Model file for the job. Use its own axes, mm. A direction names the side the tool comes from. Coordinates: 2 decimals unless noted, no trailing zeros. Write each loop counter-clockwise with the first axis right and the second up, starting at its lowest first coordinate (ties: lowest second). Pieces come first, ordered by that corner, then holes. Notation, with made-up numbers: M 76.25,-14 L 81.25,-14 A30 cw 81.25,20 Z; hole C 88.25,-6.75 d8. An arc over 180 degrees is marked long. Put each result on its own line as item: value. Start each with the question number.
Q1. Drill centre lines: line 1 along X through (y, z) = (2.3, 5); line 2 along X through (y, z) = (3.4, 8.5); line 3 along X through (y, z) = (2.7, 5). Where is each one in solid material? Low to high.
Q2. Cut at A-A (x = 0). Write the cut outline in (y, z), then the cut area to 3 significant figures.
Q3. Cut at D-D (y = 0.5). Write the cut outline in (x, z).
Q4. Drop flat-ended pins along their axis: pin 1 (0.7 mm diameter, centred on y = 3.5, z = 5, fed in from +X); pin 2 (1.5 mm diameter, centred on x = -3.5, z = 5.5, fed in from +Y); pin 3 (0.6 mm diameter, centred on x = 4, z = 2.5, fed in from +Y). Give the stop position or say it passes through.
Q5. Cut at C-C (z = 8). Write the cut outline in (x, y), then the cut area to 3 significant figures.
Q6. Which spindle directions (+Z, -Z, +X, -X, +Y, -Y) get a long thin tool onto all of the face, cutting with end or side? Do faces 1 (the flat face through (3.92, 1.46, 4.93)), 2 (the flat face through (-4, 3.3, 5)), 3 (the flat face through (4, 3.3, 5)). Say none if no direction does.
Q7. Cut at B-B (z = 5). Write the cut outline in (x, y), then the cut area to 3 significant figures.
Autodesk Inventor part; units mm, degrees
ref_plane "YZ Plane" through (0, 0, 0) normal (1, 0, 0) x (0, 1, 0)
ref_plane "XZ Plane" through (0, 0, 0) normal (0, 1, 0) x (-1, 0, 0)
ref_plane "XY Plane" through (0, 0, 0) normal (0, 0, 1) x (1, 0, 0)
sketch "Sketch_1" plane through (0, 0, 0) normal (0, 0, 1) x (1, 0, 0)
  arc A0 (-4.7999, 3.3) -> (-4.9858, 3.0264) centre (-4.7999, 3.1) ccw
  arc A1 (-4.9858, 3.0264) -> (-4.8752, 2.8208) centre (-4.056, 3.3944) ccw
  line L0 (-4.8752, 2.8208) -> (-2.9896, 0.1279)
  arc A2 (-2.9896, 0.1279) -> (-2.7438, 0) centre (-2.7438, 0.3) ccw
  line L1 (-2.7438, 0) -> (2.7438, 0)
  arc A3 (2.7438, 0) -> (2.9896, 0.1279) centre (2.7438, 0.3) ccw
  line L2 (2.9896, 0.1279) -> (4.8752, 2.8208)
  arc A4 (4.8752, 2.8208) -> (4.9858, 3.0264) centre (4.056, 3.3944) ccw
  arc A5 (4.9858, 3.0264) -> (4.7999, 3.3) centre (4.7999, 3.1) ccw
  line L3 (4.7999, 3.3) -> (2.9, 3.3)
  line L4 (2.9, 3.3) -> (2.9, 3.9)
  arc A6 (2.9, 3.9) -> (2.7, 4.1) centre (2.7, 3.9) ccw
  line L5 (2.7, 4.1) -> (-2.7, 4.1)
  arc A7 (-2.7, 4.1) -> (-2.9, 3.9) centre (-2.7, 3.9) ccw
  line L6 (-2.9, 3.9) -> (-2.9, 3.3)
  line L7 (-2.9, 3.3) -> (-4.7999, 3.3)
extrude "Extrusion1" add sketch "Sketch_1" along normal blind 10
sketch "Sketch_2" plane through (0, 0, 0) normal (1, 0, 0) x (0, 0, -1)
  line L0 (-5, 4.1) -> (-5, 0)
  line L1 (-5, 0) -> (-6.621, 0)
  line L2 (-6.621, 0) -> (-6.621, 3.721)
  line L3 (-6.621, 3.721) -> (-7, 4.1)
  line L4 (-7, 4.1) -> (-5, 4.1)
  line L5 (-5, 4.1) -> (-5, 0)
revolve "Revolution1" cut sketch "Sketch_2" angle 360 about axis through (0, 4.1, 5) along (0, 1, 0)
thread "Thread1"
properties part number "PACK-HNTT5-4"
Computed values:
1. line 1: -4.51 to -1.62, 1.62 to 4.51
1. line 2: -2.9 to 2.9
1. line 3: -4.79 to -1.62, 1.62 to 4.79
2. outline: M 0,0 L 4.1,0 L 4.1,3 L 3.72,3.38 L 0,3.38 Z; M 0,6.62 L 3.72,6.62 L 4.1,7 L 4.1,10 L 0,10 Z
2. area: 27.6 mm2
3. outline: M -3.25,0 L 3.25,0 L 3.25,10 L -3.25,10 Z; hole C 0,5 d3.24
4. pin 1: x = 4.99
4. pin 2: y = 4.09
4. pin 3: y = 3.3
5. outline: M -4.99,3.03 A1.01 ccw -4.88,2.82 L -2.99,0.13 A0.3 ccw -2.74,0 L 2.74,0 A0.3 ccw 2.99,0.13 L 4.88,2.82 A0.99 ccw 4.99,3.03 A0.2 ccw 4.8,3.3 L 2.9,3.3 L 2.9,3.9 A0.2 ccw 2.7,4.1 L -2.7,4.1 A0.2 ccw -2.9,3.9 L -2.9,3.3 L -4.8,3.3 A0.2 ccw Z
5. area: 31.3 mm2
6. face 1: +Z, -Z, +X, -Y
6. face 2: +Z, -Z, -X, +Y
6. face 3: +Z, -Z, +X, +Y
7. outline: M -4.99,3.03 A1.01 ccw -4.88,2.82 L -2.99,0.13 A0.3 ccw -2.74,0 L -1.62,0 L -1.62,3.72 L -2,4.1 L -2.7,4.1 A0.2 ccw -2.9,3.9 L -2.9,3.3 L -4.8,3.3 A0.2 ccw Z; M 1.62,0 L 2.74,0 A0.3 ccw 2.99,0.13 L 4.88,2.82 A0.99 ccw 4.99,3.03 A0.2 ccw 4.8,3.3 L 2.9,3.3 L 2.9,3.9 A0.2 ccw 2.7,4.1 L 2,4.1 L 1.62,3.72 Z
7. area: 17.9 mm2
